Model file for the job. Use its own axes, mm. A direction names the side the tool comes from. Give positions to 0.01 mm unless a question says otherwise; leave off trailing zeros. Write each loop counter-clockwise with the first axis right and the second up, starting at its lowest first coordinate (ties: lowest second). Pieces come first, ordered by that corner, then holes. Notation, with made-up numbers: (-27.75, -30) - (25.25, -30) arc R13 cw to (25.25, -23) - close; hole circle Ø6 at (88.25, 69). An arc over 180 degrees is marked (long way). Use a Markdown table: item, result. Add a question column.
```python
from build123d import *

# Parameters (mm, degrees)
BOSS_EXTRUDE2_DEPTH            = 30
BOSS_EXTRUDE2_DEPTH_BACK       = 30
EXTRUDE_THIN2_START            = -25
EXTRUDE_THIN2_DEPTH            = 50
SKETCH2_W                      = 60
SKETCH2_H                      = 5
BOSS_EXTRUDE3_DEPTH            = 100
BOSS_EXTRUDE4_DEPTH            = 30
BOSS_EXTRUDE4_DEPTH_BACK       = 30
CUT_EXTRUDE2_REACH             = 143.361
SKETCH4_W                      = 60
SKETCH4_H                      = 5
CUT_EXTRUDE2_DIRECTION_2_REACH = 143.361
BOSS_EXTRUDE5_DEPTH            = 30
BOSS_EXTRUDE5_DEPTH_BACK       = 30
DRONE_ARM_FIT_CUT_DEPTH        = 50


# Read off the part's stored shape, not the designer's step: Extrude-Thin2
with BuildPart() as part:
    # Sketch1 → Boss-Extrude2 (new, two sides: drawn at the far end of the back side and taken through both)
    with BuildSketch(Plane.XY.offset(-BOSS_EXTRUDE2_DEPTH_BACK)):
        Polygon((-13.01396445, -23.830717844), (0, -23.830717844), (0, -18.830717844), (-11.698214449, -18.830717844), (-50, 2.827283512), (-50, 13.432214294), (-55, 13.432214294), (-55, -0.089432632), align=None)
        Polygon((0, -18.830717844), (0, -23.830717844), (13.01396445, -23.830717844), (55, -0.089432632), (55, 13.432214294), (50, 13.432214294), (50, 2.827283512), (11.698214449, -18.830717844), align=None)
        with BuildLine():
            Line((-11.698214449, -18.830717844), (0, -18.830717844))
            Line((0, -18.830717844), (0, -8))
            ThreePointArc((0, -8), (-8, 0), (0, 8))
            Line((0, 8), (0, 13.432214294))
            Line((0, 13.432214294), (-50, 13.432214294))
            Line((-50, 13.432214294), (-50, 2.827283512))
            Line((-50, 2.827283512), (-11.698214449, -18.830717844))
        make_face()
        with BuildLine():
            Line((0, -8), (0, -18.830717844))
            Line((0, -18.830717844), (11.698214449, -18.830717844))
            Line((11.698214449, -18.830717844), (50, 2.827283512))
            Line((50, 2.827283512), (50, 13.432214294))
            Line((50, 13.432214294), (0, 13.432214294))
            Line((0, 13.432214294), (0, 8))
            ThreePointArc((0, 8), (5.656854249, 5.656854249), (8, 0))
            ThreePointArc((8, 0), (5.656854249, -5.656854249), (0, -8))
        make_face()
    extrude(amount=BOSS_EXTRUDE2_DEPTH + BOSS_EXTRUDE2_DEPTH_BACK)

    # Extrude-Thin2 outline → Extrude-Thin2 (add)
    with BuildSketch(Plane.XY.offset(EXTRUDE_THIN2_START)):
        Polygon((50, 13.432214294), (55, 13.432214294), (55, 68.432214294), (-55, 68.432214294), (-55, 13.432214294), (-50, 13.432214294), (-50, 63.432214294), (50, 63.432214294), align=None)
    extrude(amount=EXTRUDE_THIN2_DEPTH)

    # Sketch2 → Boss-Extrude3 (add)
    with BuildSketch(Plane.ZY.offset(-50)):
        with Locations((0, 37.694873029)):
            Rectangle(SKETCH2_W, SKETCH2_H)
    extrude(amount=BOSS_EXTRUDE3_DEPTH)

    # Sketch1<6> → Boss-Extrude4 (add, two sides: drawn at the far end of the back side and taken through both)
    with BuildSketch(Plane.XY.offset(-BOSS_EXTRUDE4_DEPTH_BACK)):
        Polygon((-55, -0.089432632), (-55, 13.432214294), (-70, 13.432214294), (-70, -8.839581066), (-16.961214453, -38.830717844), (16.961214453, -38.830717844), (70, -8.839581066), (70, 13.432214294), (55, 13.432214294), (55, -0.089432632), (13.01396445, -23.830717844), (-13.01396445, -23.830717844), align=None)
    extrude(amount=BOSS_EXTRUDE4_DEPTH + BOSS_EXTRUDE4_DEPTH_BACK)

    # Cut-Extrude2: up to this face of the body (flat: up to its plane)
    cut_extrude2_end = Plane(part.part.faces().sort_by_distance((-55, 40.932214294, 0))[0])
    # Sketch4 → Cut-Extrude2 (cut, up to the picked face)
    with BuildSketch(Plane(origin=(-50, 0, 0), x_dir=(0, 0, -1), z_dir=(1, 0, 0)), mode=Mode.PRIVATE) as cut_extrude2_sk1:
        with Locations((0, 65.932214294)):
            Rectangle(SKETCH4_W, SKETCH4_H)
    cut_extrude2_tool1 = split(extrude(cut_extrude2_sk1.sketch, amount=-CUT_EXTRUDE2_REACH, mode=Mode.PRIVATE), bisect_by=cut_extrude2_end, keep=Keep.BOTH, mode=Mode.PRIVATE)
    add(cut_extrude2_tool1.solids().sort_by(Axis((-50, 65.932214, 0), (-1, 0, 0)))[0], mode=Mode.SUBTRACT)

    # Cut-Extrude2 direction 2: up to this face of the body (flat: up to its plane)
    cut_extrude2_direction_2_end = Plane(part.part.faces().sort_by_distance((55, 40.932214294, 0))[0])
    # Sketch4 → Cut-Extrude2 direction 2 (cut, up to the picked face)
    with BuildSketch(Plane(origin=(-50, 0, 0), x_dir=(0, 0, -1), z_dir=(1, 0, 0)), mode=Mode.PRIVATE) as cut_extrude2_direction_2_sk1:
        with Locations((0, 65.932214294)):
            Rectangle(SKETCH4_W, SKETCH4_H)
    cut_extrude2_direction_2_tool1 = split(extrude(cut_extrude2_direction_2_sk1.sketch, amount=CUT_EXTRUDE2_DIRECTION_2_REACH, mode=Mode.PRIVATE), bisect_by=cut_extrude2_direction_2_end, keep=Keep.BOTH, mode=Mode.PRIVATE)
    add(cut_extrude2_direction_2_tool1.solids().sort_by(Axis((-50, 65.932214, 0), (1, 0, 0)))[0], mode=Mode.SUBTRACT)

    # Sketch1<7> → Boss-Extrude5 (add, two sides: drawn at the far end of the back side and taken through both)
    with BuildSketch(Plane.XY.offset(-BOSS_EXTRUDE5_DEPTH_BACK)):
        Polygon((-70, 13.432214294), (-55, 13.432214294), (-50, 13.432214294), (-50, 38.432214294), (-50, 63.432214294), (-70, 63.432214294), (-70, 38.432214294), align=None)
        Polygon((50, 38.432214294), (50, 13.432214294), (55, 13.432214294), (70, 13.432214294), (70, 38.432214294), (70, 63.432214294), (50, 63.432214294), align=None)
    extrude(amount=BOSS_EXTRUDE5_DEPTH + BOSS_EXTRUDE5_DEPTH_BACK)

    # Sketch7 → Drone Arm fit cut (cut)
    with BuildSketch(Plane(origin=(0, 63.432214294, 0), x_dir=(1, 0, 0), z_dir=(0, 1, 0))):
        Polygon((-70, -12.5), (-70, 12.5), (-65, 12.5), (-65, 7.5), (-60, 7.5), (-60, 12.5), (-60, 17.5), (-55, 17.5), (-55, -17.5), (-60, -17.5), (-60, -12.5), (-60, -7.5), (-65, -7.5), (-65, -12.5), align=None)
    drone_arm_fit_cut = extrude(amount=-DRONE_ARM_FIT_CUT_DEPTH, mode=Mode.SUBTRACT)

    # Mirror Drone arm fit cut: Drone Arm fit cut across plane
    add(drone_arm_fit_cut.mirror(Plane(origin=(0, 0, 0), x_dir=(0, 0, 1), z_dir=(1, 0, 0))), mode=Mode.SUBTRACT)


solid = part.part
```
(1) Band-saw the part on A-A (z = -22.5). Write the cut outline in (x, y).
(2) Band-saw the part on C-C (z = -9). Write the cut outline in (x, y).
(3) Probe probe 1 along Y at (x, z) = (-0.5, -23); probe 2 along X at (y, z) = (34, 18.5); probe 3 along Y at (x, z) = (14.5, -8.5). List the from-to ranges inside material, lowest first. Write a range as [from, to].
(4) Band-saw the part on D-D (y = -15). Write the cut outline in (x, z).
(5) Two-plate mould, pull along Z, no slides. Class faces 4 (the flat face through (58, 39, -17.5)), 5 (the flat face through (-1, 13, -30)), 6 (the flat face through (-50, 52, 0)): +Z half, -Z half, draft (parallel to the pull), parting line (faces both ways), or undercut.
(6) Band-saw the part on B-B (y = -4.5). Write the cut outline in (x, z), then the cut area to 3 significant figures.
(7) Flat gauge pins, fed straight in: pin 1 (6.5 mm diameter, centred on y = 20.5, z = 9, fed in from -X); pin 2 (6 mm diameter, centred on x = -45, z = 18.5, fed in from +Y); pin 3 (1 mm diameter, centred on y = -14, z = -14.5, fed in from +X). Where does each tip first touch, or does it go through?
(8) Which spindle directions (+Z, -Z, +X, -X, +Y, -Y) get a long thin tool onto all of the face, cutting with end or side? Do faces 1 (the flat face through (-58, 39, -17.5)), 2 (the flat face through (-63, 39, -7.5)), 3 (the flat face through (-50, 24, 0)). Say none if no direction does.
Model answer:
| question | item | result |
|---|---|---|
| 1 | outline | (-70, -8.84) - (-16.96, -38.83) - (16.96, -38.83) - (70, -8.84) - (70, 63.43) - (50, 63.43) - (50, 40.19) - (-50, 40.19) - (-50, 63.43) - (-70, 63.43) - close; hole (-50, 13.43) - (50, 13.43) - (50, 35.19) - (-50, 35.19) - close; hole circle Ø16 at (0, 0) |
| 2 | outline | (-70, -8.84) - (-16.96, -38.83) - (16.96, -38.83) - (70, -8.84) - (70, 13.43) - (65, 13.43) - (65, 63.43) - (60, 63.43) - (60, 13.43) - (55, 13.43) - (55, 63.43) - (50, 63.43) - (50, 40.19) - (-50, 40.19) - (-50, 63.43) - (-55, 63.43) - (-55, 13.43) - (-60, 13.43) - (-60, 63.43) - (-65, 63.43) - (-65, 13.43) - (-70, 13.43) - close; hole (-50, 13.43) - (50, 13.43) - (50, 35.19) - (-50, 35.19) - close; hole circle Ø16 at (0, 0) |
| 3 | probe 1 | y = [-38.83, -7.98], [7.98, 13.43], [35.19, 40.19] |
| 3 | probe 2 | x = [-70, -50], [50, 70] |
| 3 | probe 3 | y = [-38.83, 13.43], [35.19, 40.19] |
| 4 | outline | (-59.11, -30) - (59.11, -30) - (59.11, 30) - (-59.11, 30) - close |
| 5 | face 4 | undercut |
| 5 | face 5 | -Z half |
| 5 | face 6 | draft |
| 6 | outline | (-70, -30) - (-6.61, -30) - (-6.61, 30) - (-70, 30) - close; (6.61, -30) - (70, -30) - (70, 30) - (6.61, 30) - close |
| 6 | area | 7,610 mm^2 |
| 7 | pin 1 | stops at x = -65 |
| 7 | pin 2 | stops at y = 40.19 |
| 7 | pin 3 | stops at x = 61.76 |
| 8 | face 1 | +Y |
| 8 | face 2 | -X, +Y |
| 8 | face 3 | +Z, -Z |
